Verification items for the finished model (mm, model axes). Face numbers are marked on the shaded views. Give positions to 0.01 mm unless a question says otherwise; leave off trailing zeros. Order: outer loops, then holes, each group sorted by start corner. A loop starts at its lowest first (then second) coordinate and runs counter-clockwise, first axis right, second up. Notation, with made-up numbers: (-28.5, -8.5) - (-11.5, -8.5) arc R12 cw to (-11.5, -1.5) - close; hole circle Ø2 at (65, 24.25). An arc over 180 degrees is marked (long way). Answer as a JSON object with one key per item and string values.
```python
from build123d import *

# Parameters (mm, degrees)
SKETCH1_W           = 57.15
SKETCH1_H           = 64.77
SKETCH1_R           = 1.5
SKETCH1_R_2         = 3
BOSS_EXTRUDE1_DEPTH = 6.35


with BuildPart() as part:
    # Sketch1 → Boss-Extrude1 (new body)
    with BuildSketch(Plane(origin=(0, 0, 0), x_dir=(1, 0, 0), z_dir=(0, 1, 0))):
        with Locations((28.575, 32.385)):
            Rectangle(SKETCH1_W, SKETCH1_H)
        with Locations((5.08, 21.2725)):
            Circle(SKETCH1_R, mode=Mode.SUBTRACT)
        with Locations((5.08, 43.4975)):
            Circle(SKETCH1_R, mode=Mode.SUBTRACT)
        with Locations((52.07, 21.2725)):
            Circle(SKETCH1_R, mode=Mode.SUBTRACT)
        with Locations((52.07, 43.4975)):
            Circle(SKETCH1_R, mode=Mode.SUBTRACT)
        with Locations((28.575, 7.385)):
            Circle(SKETCH1_R_2, mode=Mode.SUBTRACT)
        with Locations((28.575, 57.385)):
            Circle(SKETCH1_R_2, mode=Mode.SUBTRACT)
    extrude(amount=BOSS_EXTRUDE1_DEPTH)


solid = part.part
```
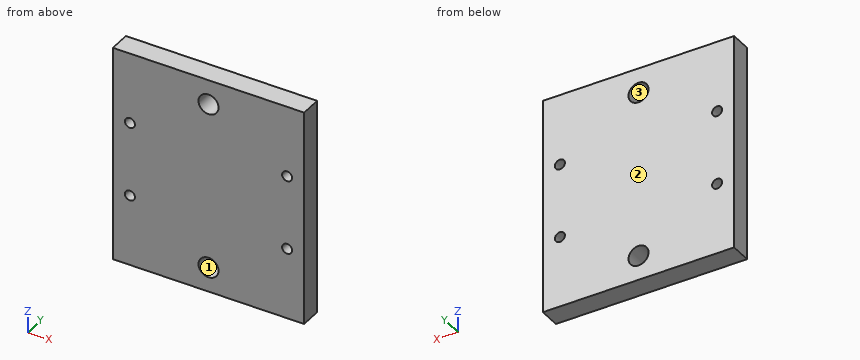
(1) Gauge pin test, flat end, axial feed: pin 1 Ø1.5 at (x, y) = (8, 2) entering from +Z. Record the tip position at first contact, or that the pin passes through.
Computed values:
{"pin 1": "stops at z = 0"}
(2) Section check A-A (x = 5.08). Record the cut outline in (y, z), then the cut area to 3 significant figures.
Computed values:
{"outline": "(0, -64.77) - (6.35, -64.77) - (6.35, -45) - (0, -45) - close; (0, -42) - (6.35, -42) - (6.35, -22.77) - (0, -22.77) - close; (0, -19.77) - (6.35, -19.77) - (6.35, 0) - (0, 0) - close", "area": "373 mm²"}
(3) Section check C-C (x = 28.5). Record the cut outline in (y, z).
Computed values:
{"outline": "(0, -64.77) - (6.35, -64.77) - (6.35, -60.38) - (0, -60.38) - close; (0, -54.39) - (6.35, -54.39) - (6.35, -10.38) - (0, -10.38) - close; (0, -4.39) - (6.35, -4.39) - (6.35, 0) - (0, 0) - close"}
(4) Release check for a two-part mould opening along X. For the marked faces 1, 2 and 3 record: pulls with the +X half, pulls with the -X half, needs draft (parallel to the pull), parting line crosses it, or undercut.
Computed values:
{"face 1": "undercut", "face 2": "needs draft", "face 3": "undercut"}
(5) Material ranges on line 1 along X through (y, z) = (3, -43.5); line 2 along Z through (x, y) = (52.07, 1.75); line 3 along X through (y, z) = (1.5, -22.5), recorded low to high. Write a range as [from, to].
Computed values:
{"line 1": "x = [0, 3.58], [6.58, 50.57], [53.57, 57.15]", "line 2": "z = [-64.77, -45], [-42, -22.77], [-19.77, 0]", "line 3": "x = [0, 4.22], [5.94, 51.21], [52.93, 57.15]"}
(6) Section check B-B (y = 0.75). Count the separate pieces of the cut face and the enclosed holes in it, then the cut area to 3 significant figures.
Computed values:
{"separate pieces": "1", "enclosed holes": "6", "area": "3,620 mm²"}
